Design review of the part built by this model. Coordinates are the model's own, in mm. A direction names the side the tool comes from. Coordinates: 2 decimals unless noted, no trailing zeros. Loops run counter-clockwise (first coordinate to the right, second up) from the corner with the lowest first, then second, coordinate; pieces in that order, holes last. Notation, with made-up numbers: (65, 76.5) -> (93, 76.5) arc R23 cw to (93, 104.5) -> close; hole circle Ø11 at (77, -29.75). An arc over 180 degrees is marked (long way). Use a Markdown table: item, result. Add a question column.
Q1. Take a section at C-C on x = 0. Write out the cut boundary in (y, z), plus the area to 3 significant figures.
Q2. For probe 1 along Z at (x, y) = (0, -0.4); probe 2 along X at (y, z) = (-2, 50.5); probe 3 along Z at (x, y) = (-12, 2), list the stretches that pass through material, from the lowest coordinate up.
Q3. Draft analysis for pull direction Z (two halves, no side actions). For faces 1 (the face through (-0.54, -0.04, 52.56)), 2 (the face through (0, -2.5, 42)), 3 (the face through (0, -5, 25)), state which applies: pulls with the +Z half, pulls with the -Z half, needs draft (parallel to the pull), parting line crosses it, or undercut.
Q4. Clearance check with flat-ended pins moving along their axes: pin 1 Ø1 at (x, y) = (-15.5, -1) entering from +Z; pin 2 Ø2 at (y, z) = (-18.5, 23.5) entering from +X; pin 3 Ø6 at (x, z) = (14.5, -14.5) entering from -Y. State where each tip first meets the part, or that it passes through.
Q5. Take a section at B-B on y = 0. Write out the cut boundary in (x, z), plus the area to 3 significant figures.
Q6. Take a section at A-A on z = 53.5. Write out the cut boundary in (x, y), plus the area to 3 significant figures.
Q7. For faces 4 (the face through (0, 2.5, 42)), 5 (the face through (-7.5, 0, 41)), 6 (the face through (7.5, 0, 41)), list the 3-axis set-ups (+Z, -Z, +X, -X, +Y, -Y) from which the entire face can be reached by the end or side of a thin tool; tool diameter is ignored.
Q8. Take a section at D-D on z = -17. Write out the cut boundary in (x, y).
from build123d import *

# Parameters (mm, degrees)
F0_R     = 25
F1_DEPTH = 25
F2_W     = 15
F2_H     = 5
F3_DEPTH = 35
F4_R     = 2.5
F5_DEPTH = 5
F6_SIZE  = 3


with BuildPart() as f1:
    # F0 (on Top) → F1 (new body, symmetric)
    with BuildSketch(Plane.XY):
        Circle(F0_R)
    extrude(amount=F1_DEPTH, both=True)

    # F2 (on face) → F3 (join)
    with BuildSketch(Plane.XY.offset(25)):
        Rectangle(F2_W, F2_H)
    extrude(amount=F3_DEPTH)

    # F4 (on face) → F5 (cut, through all)
    with BuildSketch(Plane.XZ.offset(2.5)):
        with Locations((0, 55)):
            Circle(F4_R)
    extrude(amount=-F5_DEPTH, mode=Mode.SUBTRACT)

    # F6
    f6_edges = [f1.edges().sort_by_distance(p)[0] for p in [
        (-25, 0, 25),
        (-25, 0, -25),
        (-7.5, 0, 60),
        (7.5, 0, 60),
    ]]
    chamfer(f6_edges, length=F6_SIZE)


solid = f1.part
Answer list:
| question | item | result |
|---|---|---|
| 1 | outline | (-25, -22) -> (-22, -25) -> (22, -25) -> (25, -22) -> (25, 22) -> (22, 25) -> (2.5, 25) -> (2.5, 52.5) -> (-2.5, 52.5) -> (-2.5, 25) -> (-22, 25) -> (-25, 22) -> close; (-2.5, 57.5) -> (2.5, 57.5) -> (2.5, 60) -> (-2.5, 60) -> close |
| 1 | area | 2,630 mm² |
| 2 | probe 1 | -25 to 52.5, 57.5 to 60 |
| 2 | probe 2 | -7.5 to 7.5 |
| 2 | probe 3 | -25 to 25 |
| 3 | face 1 | undercut |
| 3 | face 2 | needs draft |
| 3 | face 3 | pulls with the +Z half |
| 4 | pin 1 | z = 25 |
| 4 | pin 2 | x = 16.43 |
| 4 | pin 3 | y = -22.2 |
| 5 | outline | (-25, -22) -> (-22, -25) -> (22, -25) -> (25, -22) -> (25, 22) -> (22, 25) -> (7.5, 25) -> (7.5, 57) -> (4.5, 60) -> (-4.5, 60) -> (-7.5, 57) -> (-7.5, 25) -> (-22, 25) -> (-25, 22) -> close; hole circle Ø5 at (0, 55) |
| 5 | area | 2,980 mm² |
| 6 | outline | (-7.5, -2.5) -> (-2, -2.5) -> (-2, 2.5) -> (-7.5, 2.5) -> close; (2, -2.5) -> (7.5, -2.5) -> (7.5, 2.5) -> (2, 2.5) -> close |
| 6 | area | 55.0 mm² |
| 7 | face 4 | +Z, +X, -X, +Y |
| 7 | face 5 | +Z, -X, +Y, -Y |
| 7 | face 6 | +Z, +X, +Y, -Y |
| 8 | outline | circle Ø50 at (0, 0) |
